from build123d import *

# Parameters (mm, degrees)
F1_DEPTH = 10.033
F3_DEPTH = 76.2
F5_DEPTH = 76.2
F7_D     = 2.921
F7_DEPTH = 8.255
F9_DEPTH = 4.446


with BuildPart() as f1:
    # F0 (on Right) → F1 (new body, symmetric)
    with BuildSketch(Plane.YZ):
        Polygon((19.05, -6.35), (31.75, 6.35), (-19.05, 6.35), (-31.75, -6.35), align=None)
    extrude(amount=F1_DEPTH, both=True)

    # F2 (on Front) → F3 (cut, symmetric)
    with BuildSketch(Plane.XZ):
        Polygon((-6.858, -3.81), (-5.588, -6.35), (5.588, -6.35), (6.858, -3.81), align=None)
        Polygon((5.588, 6.35), (-5.588, 6.35), (-6.858, 3.81), (6.858, 3.81), align=None)
    extrude(amount=F3_DEPTH, both=True, mode=Mode.SUBTRACT)

    # F4 (on Front) → F5 (cut, symmetric)
    with BuildSketch(Plane.XZ):
        Polygon((16.257983, -9.573173), (10.033, 0), (5.588, 0), (5.588, 6.35), (-11.387688, 6.35), (-11.387688, -9.573173), align=None)
    extrude(amount=F5_DEPTH, both=True, mode=Mode.SUBTRACT)

    # F7
    with Locations(Plane(origin=(5.588, 0, 0), x_dir=(0, -1, 0), z_dir=(-1, 0, 0))):
        with Locations((-15.875, 1.905), (9.525, 1.905)):
            Hole(F7_D / 2, depth=F7_DEPTH)

    # F8 (on face) → F9 (cut, through all)
    with BuildSketch(Plane.YZ.offset(10.033)):
        Polygon((-19.05, 6.35), (-25.4, 0), (-19.05, 0), align=None)
        Polygon((25.4, 6.35), (25.4, 0), (31.75, 6.35), align=None)
    extrude(amount=-F9_DEPTH, mode=Mode.SUBTRACT)


solid = f1.part
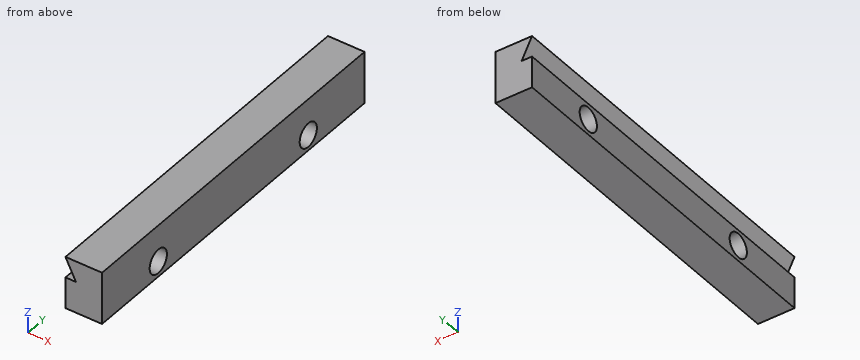
Geometry check sheet. Reference: the model listing, model coordinates, mm. Give positions to 0.01 mm unless a question says otherwise; leave off trailing zeros. Loops run counter-clockwise (first coordinate to the right, second up) from the corner with the lowest first, then second, coordinate; pieces in that order, holes last. Notation, with made-up numbers: (37, -31.5) -> (85, -31.5) arc R17 ccw to (85, -25.5) -> close; hole circle Ø3 at (50.5, 69). An arc over 180 degrees is marked (long way). Answer in a Markdown table with one row per item. Add a question column.
1) Cross-section at C-C on y = 22.5. Record the boundary of the cut face in (x, z), and give its area (3 significant figures).
2) Gauge pin test, flat end, axial feed: P1, Ø2.5, axis at y = -9.525, z = 1.905, coming from the +X side. Record the tip position at first contact, or that the pin passes through.
3) Cross-section at B-B on z = 1.5. Record the boundary of the cut face in (x, y), and give its area (3 significant figures).
4) Cross-section at A-A on x = 6.4. State how many separate pieces and enclosed holes the cut face has, and give its area (3 significant figures).
5) Material ranges on probe 1 along Y at (x, z) = (7.2, 1.75); probe 2 along Y at (x, z) = (8.65, 2.75); probe 3 along Z at (x, y) = (6.15, 8.5), recorded low to high. Write a range as from..to.
Outcome:
| question | item | result |
|---|---|---|
| 1 | outline | (5.59, 0) -> (10.03, 0) -> (10.03, 6.35) -> (5.59, 6.35) -> (6.86, 3.81) -> (5.59, 3.81) -> close |
| 1 | area | 26.6 mm^2 |
| 2 | P1 | passes through |
| 3 | outline | (5.59, -19.05) -> (10.03, -19.05) -> (10.03, -10.93) -> (5.59, -10.93) -> close; (5.59, -8.12) -> (10.03, -8.12) -> (10.03, 14.47) -> (5.59, 14.47) -> close; (5.59, 17.28) -> (10.03, 17.28) -> (10.03, 25.4) -> (5.59, 25.4) -> close |
| 3 | area | 173 mm^2 |
| 4 | separate pieces | 2 |
| 4 | enclosed holes | 2 |
| 4 | area | 228 mm^2 |
| 5 | probe 1 | y = -19.05..-10.98, -8.07..14.42, 17.33..25.4 |
| 5 | probe 2 | y = -19.05..-10.72, -8.33..14.68, 17.07..25.4 |
| 5 | probe 3 | z = 0..3.81, 5.23..6.35 |
